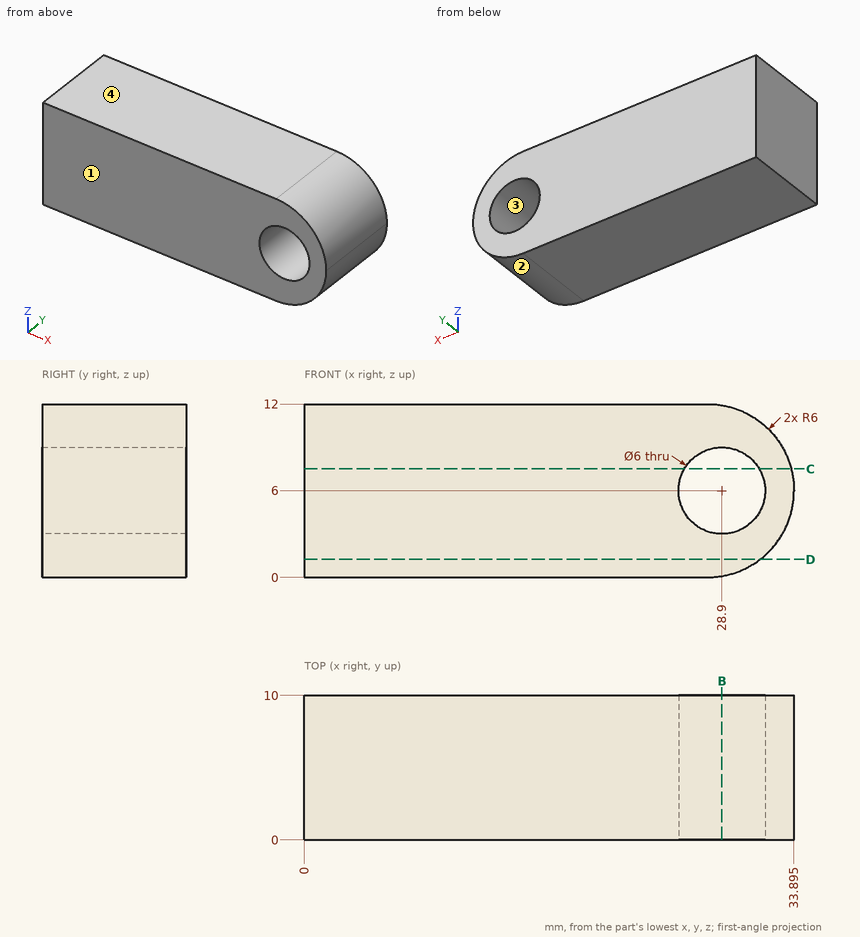
Study the drawing (mm; zero at the part's minimum x, y, z) and answer. Give positions to 0.01 mm unless a question says otherwise; leave off trailing zeros. Write each loop counter-clockwise with the first axis right and the second up, starting at its lowest first coordinate (ties: lowest second). Pieces come first, ordered by that corner, then holes. Notation, with made-up numbers: (42.5, 12.25) -> (64.5, 12.25) arc R27 cw to (64.5, 45.25) -> close; hole circle Ø6 at (42.5, 12.5). An arc over 180 degrees is marked (long way). Answer as a JSON object with one key per item and string values. Group by question number.
1) Find section D-D (z = 1.25). Write down the section's boundary in (x, y).
2) Consider L1, parallel to X at y = 7, z = 6 (1 decimal); L2, parallel to X at y = 7.5, z = 6.75 (1 decimal); L3, parallel to X at y = 1, z = 2.5. Determine where each line is inside the solid, lowest interval first. Write a range as from..to.
3) Find section B-B (x = 28.9). Write down the section's boundary in (y, z) (1 decimal).
4) Find section C-C (z = 7.5). Write down the section's boundary in (x, y) (1 decimal).
5) The mould has two halves that part along Z. Classify the marked faces 1, 2, 3 and 4: +Z half, -Z half, draft (parallel to the pull), parting line (faces both ways), or undercut.
Values follow:
{
 "1": {"outline": "(0, 0) -> (31.56, 0) -> (31.56, 10) -> (0, 10) -> close"},
 "2": {"L1": "x = 0..25.9, 31.9..33.9", "L2": "x = 0..26, 31.8..33.8", "L3": "x = 0..32.77"},
 "3": {"outline": "(0, 0.1) -> (10, 0.1) -> (10, 3) -> (0, 3) -> close; (0, 9) -> (10, 9) -> (10, 11.9) -> (0, 11.9) -> close"},
 "4": {"outline": "(0, 0) -> (26.3, 0) -> (26.3, 10) -> (0, 10) -> close; (31.5, 0) -> (33.7, 0) -> (33.7, 10) -> (31.5, 10) -> close"},
 "5": {"face 1": "draft", "face 2": "-Z half", "face 3": "undercut", "face 4": "+Z half"}
}
